CAD build for the part. Positions are in the model's coordinates, mm. Face numbers are marked on the shaded views. A direction names the side the tool comes from. Give positions to 0.01 mm unless a question says otherwise; leave off trailing zeros. Loops run counter-clockwise (first coordinate to the right, second up) from the corner with the lowest first, then second, coordinate; pieces in that order, holes last. Notation, with made-up numbers: M -32.5,80.5 L 18.5,80.5 A5 cw 18.5,84.5 Z; hole C -22,71 d9. An arc over 180 degrees is marked long. Answer as CSV lines item,"result".
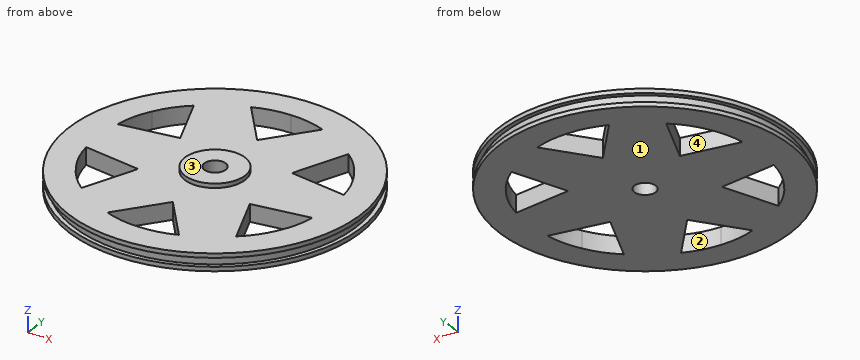
```python
from build123d import *

# Parameters (mm, degrees)
SKETCH1_R           = 67.5
SKETCH1_R_2         = 5
BOSS_EXTRUDE1_DEPTH = 4
CUT_EXTRUDE1_DEPTH  = 4
CIRPATTERN1_COUNT   = 6
SKETCH3_R           = 67.5
SKETCH3_R_2         = 65.5
CUT_EXTRUDE2_DEPTH  = 2
SKETCH4_R           = 13.962380749
SKETCH4_R_2         = 5
BOSS_EXTRUDE2_DEPTH = 2


with BuildPart() as part:
    # Sketch1 → Boss-Extrude1 (new, symmetric)
    with BuildSketch(Plane.XY):
        Circle(SKETCH1_R)
        Circle(SKETCH1_R_2, mode=Mode.SUBTRACT)
    extrude(amount=BOSS_EXTRUDE1_DEPTH, both=True)

    # Sketch2 → Cut-Extrude1 (cut, symmetric)
    with BuildSketch(Plane.XY):
        with BuildLine():
            Line((0, 30.239217172), (-16.768164039, 51.529133311))
            ThreePointArc((-16.768164039, 51.529133311), (-8.53840593, 53.919450475), (0, 54.653043584))
            ThreePointArc((0, 54.653043584), (8.53840593, 53.919450475), (16.768164039, 51.529133311))
            Line((16.768164039, 51.529133311), (0, 30.239217172))
        make_face()
    cut_extrude1 = extrude(amount=CUT_EXTRUDE1_DEPTH, both=True, mode=Mode.SUBTRACT)

    # CirPattern1: Cut-Extrude1 ×6 about axis
    cirpattern1_axis = Axis((0, 0, 0), (0, 0, 1))
    for i in range(1, CIRPATTERN1_COUNT):
        add(cut_extrude1.rotate(cirpattern1_axis, i * 360 / CIRPATTERN1_COUNT), mode=Mode.SUBTRACT)

    # Sketch3 → Cut-Extrude2 (cut, symmetric)
    with BuildSketch(Plane.XY):
        Circle(SKETCH3_R)
        Circle(SKETCH3_R_2, mode=Mode.SUBTRACT)
    extrude(amount=CUT_EXTRUDE2_DEPTH, both=True, mode=Mode.SUBTRACT)

    # Sketch4 → Boss-Extrude2 (add)
    with BuildSketch(Plane.XY.offset(4)):
        Circle(SKETCH4_R)
        Circle(SKETCH4_R_2, mode=Mode.SUBTRACT)
    extrude(amount=BOSS_EXTRUDE2_DEPTH)


solid = part.part
```
Q1. Which spindle directions (+Z, -Z, +X, -X, +Y, -Y) get a long thin tool onto all of the face, cutting with end or side? Do the marked faces 3 and 4. Say none if no direction does.
Solution:
face 3,"+Z, +X, -X, +Y, -Y"
face 4,"+Z, -Z"
Q2. Cut at D-D (x = 10). Write the cut outline in (y, z).
Solution:
outline,"M -66.76,-4 L -53.62,-4 L -53.62,4 L -66.76,4 L -66.76,2 L -64.73,2 L -64.73,-2 L -66.76,-2 Z; M -42.94,-4 L 42.94,-4 L 42.94,4 L 9.74,4 L 9.74,6 L -9.74,6 L -9.74,4 L -42.94,4 Z; M 53.62,-4 L 66.76,-4 L 66.76,-2 L 64.73,-2 L 64.73,2 L 66.76,2 L 66.76,4 L 53.62,4 Z"
Q3. Mould opens along X. For the marked faces 1 and 2 say: released by +X, released by -X, zero draft, split by the parting line, or undercut.
Solution:
face 1,"zero draft"
face 2,"undercut"
Q4. Cut at A-A (y = 0). Write the cut outline in (x, z), and give its area (3 significant figures).
Solution:
outline,"M -67.5,-4 L -5,-4 L -5,6 L -13.96,6 L -13.96,4 L -67.5,4 L -67.5,2 L -65.5,2 L -65.5,-2 L -67.5,-2 Z; M 5,-4 L 67.5,-4 L 67.5,-2 L 65.5,-2 L 65.5,2 L 67.5,2 L 67.5,4 L 13.96,4 L 13.96,6 L 5,6 Z"
area,"1,020 mm²"
Q5. Pin check, flat tips, straight feed: P1, Ø1.5, axis at y = 50, z = -0.5, coming from the -X side; P2, Ø1, axis at x = -43.5, y = -14.5, coming from the -Z side; P3, Ø8, axis at x = -36.5, y = -15.5, coming from the +Z side; P4, Ø4, axis at y = 43.5, z = 1.5, coming from the +X side. Stop position of each tip, or through.
Solution:
P1,"stops at x = -43.18"
P2,"passes through"
P3,"stops at z = 4"
P4,"stops at x = 53.19"
Q6. Cut at C-C (y = -17). Write the cut outline in (x, z).
Solution:
outline,"M -65.32,-4 L -51.78,-4 L -51.78,4 L -65.32,4 L -65.32,2 L -63.26,2 L -63.26,-2 L -65.32,-2 Z; M -26.94,-4 L 26.94,-4 L 26.94,4 L -26.94,4 Z; M 51.78,-4 L 65.32,-4 L 65.32,-2 L 63.26,-2 L 63.26,2 L 65.32,2 L 65.32,4 L 51.78,4 Z"
Q7. Cut at B-B (x = -12). Write the cut outline in (y, z), and give its area (3 significant figures).
Solution:
outline,"M -66.42,-4 L -53.13,-4 L -53.13,4 L -66.42,4 L -66.42,2 L -64.39,2 L -64.39,-2 L -66.42,-2 Z; M -45.48,-4 L 45.48,-4 L 45.48,4 L 7.14,4 L 7.14,6 L -7.14,6 L -7.14,4 L -45.48,4 Z; M 53.13,-4 L 66.42,-4 L 66.42,-2 L 64.39,-2 L 64.39,2 L 66.42,2 L 66.42,4 L 53.13,4 Z"
area,"953 mm²"
Q8. Wall check: line 1 (Y direction, x = -43.5, z = -0.5); line 2 (X direction, y = -32, z = -0.5); line 3 (Y direction, x = 41, z = -1.75). Give the ranges that are in metal, low to high. Write a range as [from, to].
Solution:
line 1,"y = [-48.97, -33.05], [-12.62, 12.62], [33.05, 48.97]"
line 2,"x = [-57.15, -44.3], [-32.93, -1.39], [1.39, 32.93], [44.3, 57.15]"
line 3,"y = [-51.08, -35.94], [-12.98, 12.98], [35.94, 51.08]"
